Read the model definition and answer for the solid it produces. Units are mm, in the model's axes. A direction names the side the tool comes from. Give positions to 0.01 mm unless a question says otherwise; leave off trailing zeros. Order: outer loops, then holes, each group sorted by start corner. A loop starts at its lowest first (then second) coordinate and runs counter-clockwise, first axis right, second up.
Item 1: A cutting plane is placed at A-A (y = 0). Write down the section's boundary in (x, z), plus the area to 3 significant figures.
Item 2: Which of the six approach directions +Z, -Z, +X, -X, +Y, -Y give full straight-line access (tool end or side, diameter ignored) to faces 1 (the face through (-1.38, -6.2, 25.31)), 2 (the face through (123.98, -27.53, 9.64))?
Item 3: Find the intervals of material crossed by line 1 along Z through (x, y) = (-34, 23); line 2 along X through (y, z) = (-53, 6); line 3 along Y through (x, z) = (-76, 14.5), in increasing order.
Item 4: Given pin 1 Ø10 at (x, z) = (32.5, 21.5) entering from -Y; pin 2 Ø5 at (x, y) = (-12.5, 61.5) entering from +Z; pin 3 Ø1.5 at (y, z) = (-90.5, 11.5) entering from +X, each flat-ended and moving along its own axis, determine where each tip first touches the part or whether it passes through.
Item 5: A cutting plane is placed at C-C (z = 6.5). Write down the section's boundary in (x, y), plus the area to 3 significant figures.
from build123d import *

# Parameters (mm, degrees)
F0_W     = 127
F0_H     = 19.05
F2_SIZE2 = 1.5875
F2_SIZE  = 1.5875
F3_R     = 6.35
F4_DEPTH = 12.7


with BuildPart() as f1:
    # F0 (on Right) → F1 (revolve)
    with BuildSketch(Plane.YZ):
        with Locations((63.5, 9.525)):
            Rectangle(F0_W, F0_H)
    revolve(axis=Axis((0, 0, 9.525), (0, 0, 1)))

    # F2
    f2_edges = [f1.edges().sort_by_distance(p)[0] for p in [
        (0, -127, 0),
        (0, -127, 19.05),
    ]]
    chamfer(f2_edges, length=F2_SIZE, length2=F2_SIZE2)

    # F3 (on face) → F4 (join)
    with BuildSketch(Plane.XY.offset(19.05)):
        Circle(F3_R)
    extrude(amount=F4_DEPTH)


solid = f1.part
Response values:
1. outline: (-127, 1.59) - (-125.41, 0) - (125.41, 0) - (127, 1.59) - (127, 17.46) - (125.41, 19.05) - (6.35, 19.05) - (6.35, 31.75) - (-6.35, 31.75) - (-6.35, 19.05) - (-125.41, 19.05) - (-127, 17.46) - close
1. area: 4,990 mm2
2. face 1: +Z
2. face 2: +Z, -Z
3. line 1: z = 0 to 19.05
3. line 2: x = -115.41 to 115.41
3. line 3: y = -101.75 to 101.75
4. pin 1: stops at y = -123.51
4. pin 2: stops at z = 19.05
4. pin 3: stops at x = 89.86
5. outline: circle Ø254 at (0, 0)
5. area: 50,700 mm2
